```python
from build123d import *

# Parameters (mm, degrees)
SKETCH2_R               = 1.5875
EXTRUDE1_DEPTH          = 25.4
EXTRUDE1_DEPTH_BACK     = 25.4
CHAMFER1_SIZE           = 0.3175
SKETCH3_OUTSIDE_W       = 15.376
SKETCH3_OUTSIDE_H       = 15.376
SKETCH3_OUTSIDE_R       = 1.4859
CUT_EXTRUDE1_DEPTH      = 0.3048
SKETCH4_OUTSIDE_W       = 15.376
SKETCH4_OUTSIDE_H       = 15.376
SKETCH4_OUTSIDE_R       = 1.4859
CUT_EXTRUDE2_DEPTH      = 0.3048
SKETCH5_W               = 17.4752
SKETCH5_H               = 6.35
SKETCH5_W_2             = 1.6002
CUT_EXTRUDE3_DEPTH      = 2.5875
CUT_EXTRUDE3_DEPTH_BACK = 2.5875


with BuildPart() as part:
    # Sketch2 → Extrude1 (new body, two sides)
    with BuildSketch(Plane(origin=(0, 0, 0), x_dir=(0, 0, -1), z_dir=(1, 0, 0))) as extrude1_sk:
        Circle(SKETCH2_R)
    extrude(amount=EXTRUDE1_DEPTH)
    extrude(extrude1_sk.sketch, amount=-EXTRUDE1_DEPTH_BACK)

    # Chamfer1
    chamfer1_edges = [part.edges().sort_by_distance(p)[0] for p in [
        (-25.4, 0, 1.5875),
        (25.4, 0, 1.5875),
    ]]
    chamfer(chamfer1_edges, length=CHAMFER1_SIZE)

    # Sketch3 outside → Cut-Extrude1 (cut)
    with BuildSketch(Plane.ZY.offset(22.225)):
        Rectangle(SKETCH3_OUTSIDE_W, SKETCH3_OUTSIDE_H)
        Circle(SKETCH3_OUTSIDE_R, mode=Mode.SUBTRACT)
    extrude(amount=CUT_EXTRUDE1_DEPTH, mode=Mode.SUBTRACT)

    # Sketch4 outside → Cut-Extrude2 (cut)
    with BuildSketch(Plane.ZY.offset(-6.35)):
        Rectangle(SKETCH4_OUTSIDE_W, SKETCH4_OUTSIDE_H)
        Circle(SKETCH4_OUTSIDE_R, mode=Mode.SUBTRACT)
    extrude(amount=-CUT_EXTRUDE2_DEPTH, mode=Mode.SUBTRACT)

    # Sketch5 → Cut-Extrude3 (cut, two sides)
    with BuildSketch(Plane.XY) as cut_extrude3_sk:
        with Locations((16.6624, 0)):
            Rectangle(SKETCH5_W, SKETCH5_H)
        with Locations((-24.5999, 0)):
            Rectangle(SKETCH5_W_2, SKETCH5_H)
    extrude(amount=CUT_EXTRUDE3_DEPTH, mode=Mode.SUBTRACT)
    extrude(cut_extrude3_sk.sketch, amount=-CUT_EXTRUDE3_DEPTH_BACK, mode=Mode.SUBTRACT)


solid = part.part
```
CAD build for the part. Positions are in the model's coordinates, mm. A direction names the side the tool comes from. Give positions to 0.01 mm unless a question says otherwise; leave off trailing zeros. Loops run counter-clockwise (first coordinate to the right, second up) from the corner with the lowest first, then second, coordinate; pieces in that order, holes last. Notation, with made-up numbers: (15, 75) -> (50, 75) arc R18 cw to (50, 89) -> close; hole circle Ø2 at (41.25, 50.5). An arc over 180 degrees is marked (long way). Use a Markdown table: item, result.
1. Mould opens along X. For faces 3 (the cylindrical face through (-22.375, 0.446, 1.417)), 4 (the flat face through (-23.8, 0, 0)), 5 (the cylindrical face through (7.3, -1.55, 0.34)) say: pulls with the +X half, pulls with the -X half, needs draft (parallel to the pull), parting line crosses it, or undercut.
Check result:
| item | result |
|---|---|
| face 3 | undercut |
| face 4 | pulls with the -X half |
| face 5 | needs draft |
2. Flat gauge pin, fed straight in: pin 1 (1.5 mm diameter, centred on x = -5.5, y = 1, fed in from -Z). Where does the tip first touch, or does it go through?
Check result:
| item | result |
|---|---|
| pin 1 | stops at z = -1.57 |
3. Which spindle directions (+Z, -Z, +X, -X, +Y, -Y) get a long thin tool onto all of the face, cutting with end or side? Do faces 1 (the cylindrical face through (6.5, 0.446, 1.417)), 2 (the cylindrical face through (-23.16, -1.55, 0.34)). Say none if no direction does.
Check result:
| item | result |
|---|---|
| face 1 | none |
| face 2 | +X, -X |
4. Slice it at C-C (x = 0.5). List the corners of the cut face in (y, z) (1 decimal).
Check result:
| item | result |
|---|---|
| outline | circle Ø3.2 at (0, 0) |
5. Slice it at B-B (y = 0.7). List the corners of the cut face in (x, z) (3 decimals).
Check result:
| item | result |
|---|---|
| outline | (-23.8, -1.425) -> (-22.53, -1.425) -> (-22.53, -1.311) -> (-22.225, -1.311) -> (-22.225, -1.425) -> (6.35, -1.425) -> (6.35, -1.311) -> (6.655, -1.311) -> (6.655, -1.425) -> (7.925, -1.425) -> (7.925, 1.425) -> (6.655, 1.425) -> (6.655, 1.311) -> (6.35, 1.311) -> (6.35, 1.425) -> (-22.225, 1.425) -> (-22.225, 1.311) -> (-22.53, 1.311) -> (-22.53, 1.425) -> (-23.8, 1.425) -> close |
6. Wall check: L1, parallel to Z at x = -21, y = 0.1; L2, parallel to Y at x = 4, z = -0.2; L3, parallel to Z at x = -16.5, y = 0.9. Give the ranges that are in metal, low to high. Write a range as [from, to].
Check result:
| item | result |
|---|---|
| L1 | z = [-1.58, 1.58] |
| L2 | y = [-1.57, 1.57] |
| L3 | z = [-1.31, 1.31] |
7. Slice it at A-A (z = 0.75). List the corners of the cut face in (x, y) (3 decimals), plus the area to 3 significant figures.
Check result:
| item | result |
|---|---|
| outline | (-23.8, -1.399) -> (-22.53, -1.399) -> (-22.53, -1.283) -> (-22.225, -1.283) -> (-22.225, -1.399) -> (6.35, -1.399) -> (6.35, -1.283) -> (6.655, -1.283) -> (6.655, -1.399) -> (7.925, -1.399) -> (7.925, 1.399) -> (6.655, 1.399) -> (6.655, 1.283) -> (6.35, 1.283) -> (6.35, 1.399) -> (-22.225, 1.399) -> (-22.225, 1.283) -> (-22.53, 1.283) -> (-22.53, 1.399) -> (-23.8, 1.399) -> close |
| area | 88.6 mm^2 |
